from build123d import *

# Parameters (mm, degrees)
CROQUIS1_W                                           = 98
CROQUIS1_H                                           = 80
SALIENTE_EXTRUIR1_DEPTH                              = 200
VACIADO1_T                                           = -5
REDONDEO1_R                                          = 2
CROQUIS6_R                                           = 4.5
CORTAR_EXTRUIR3_DEPTH                                = 401.03249868
REFRENTADO_PARA_TORNILLO_CON_CABEZA_PLAN_D           = 3.4
REFRENTADO_PARA_TORNILLO_CON_CABEZA_PLAN_DEPTH       = 5
REFRENTADO_PARA_TORNILLO_CON_CABEZA_PLAN_CBORE_D     = 6.5
REFRENTADO_PARA_TORNILLO_CON_CABEZA_PLAN_CBORE_DEPTH = 2
CORTAR_EXTRUIR5_REACH                                = 228.283
CROQUIS11_R                                          = 6.5
SIMETR_A3_AT_THE_SECOND_PLANE_COPY_1_REACH           = 228.283
SIMETR_A3_AT_THE_SECOND_PLANE_COPY_1_SKE_R           = 6.5
REFRENTADO_PARA_TORNILLO_CON_CABEZA_2_D              = 3.4
REFRENTADO_PARA_TORNILLO_CON_CABEZA_2_DEPTH          = 5
REFRENTADO_PARA_TORNILLO_CON_CABEZA_2_CBORE_D        = 6.5
REFRENTADO_PARA_TORNILLO_CON_CABEZA_2_CBORE_DEPTH    = 2
REFRENTADO_PARA_TORNILLO_CON_CABEZA_3_D              = 3.4
REFRENTADO_PARA_TORNILLO_CON_CABEZA_3_DEPTH          = 5
REFRENTADO_PARA_TORNILLO_CON_CABEZA_3_CBORE_D        = 6.5
REFRENTADO_PARA_TORNILLO_CON_CABEZA_3_CBORE_DEPTH    = 2
REFRENTADO_PARA_TORNILLO_CON_CABEZA_4_D              = 3.2
REFRENTADO_PARA_TORNILLO_CON_CABEZA_4_DEPTH          = 5
REFRENTADO_PARA_TORNILLO_CON_CABEZA_4_CBORE_D        = 6.5
REFRENTADO_PARA_TORNILLO_CON_CABEZA_4_CBORE_DEPTH    = 2
CROQUIS21_W                                          = 20.5
CROQUIS21_H                                          = 41
CORTAR_EXTRUIR6_DEPTH                                = 10
SALIENTE_EXTRUIR2_DEPTH                              = 42.5
CORTAR_EXTRUIR7_REACH                                = 222.909
CROQUIS24_W                                          = 85
CROQUIS24_H                                          = 221.577794898
SALIENTE_EXTRUIR7_DEPTH                              = 4
CORTAR_EXTRUIR8_REACH                                = 230.263
TALADRO_DE_MARGEN_PARA_M31_D                         = 3.4
TALADRO_DE_MARGEN_PARA_M31_DEPTH                     = 5
TALADRO_DE_MARGEN_PARA_M51_D                         = 5.5
TALADRO_DE_MARGEN_PARA_M51_DEPTH                     = 5
CROQUIS30_W                                          = 10
CROQUIS30_H                                          = 10
SALIENTE_EXTRUIR8_DEPTH                              = 5
TALADRO_DE_MARGEN_PARA_M52_D                         = 5.5
TALADRO_DE_MARGEN_PARA_M52_DEPTH                     = 5


with BuildPart() as part:
    # Croquis1 → Saliente-Extruir1 (new, symmetric)
    with BuildSketch(Plane.XY):
        Rectangle(CROQUIS1_W, CROQUIS1_H)
    extrude(amount=SALIENTE_EXTRUIR1_DEPTH, both=True)

    # Vaciado1
    vaciado1_openings = [part.faces().sort_by_distance(p)[0] for p in [
        (0, 40, 0),
    ]]
    offset(amount=VACIADO1_T, openings=vaciado1_openings, kind=Kind.INTERSECTION)

    # Redondeo1
    redondeo1_edges = [part.edges().sort_by_distance(p)[0] for p in [
        (49, 0, 200),
        (0, -35, -195),
        (0, -35, 195),
        (-49, 0, 200),
        (49, 0, -200),
        (0, -40, -200),
        (-49, 0, -200),
        (49, 40, 0),
        (49, -40, 0),
        (-49, -40, 0),
        (0, -40, 200),
    ]]
    fillet(redondeo1_edges, radius=REDONDEO1_R)

    # Croquis6 → Cortar-Extruir3 (cut, through all)
    with BuildSketch(Plane(origin=(0, 0, 195), x_dir=(-1, 0, 0), z_dir=(0, 0, -1))):
        with Locations((1, 20)):
            Circle(CROQUIS6_R)
    extrude(amount=-CORTAR_EXTRUIR3_DEPTH, mode=Mode.SUBTRACT)

    # Refrentado para tornillo con cabeza plan
    with Locations(Plane.ZY.offset(49)):
        with Locations((-184, -27.06), (-184, -9.06), (-151, -9.06), (-151, -27.06)):
            CounterBoreHole(REFRENTADO_PARA_TORNILLO_CON_CABEZA_PLAN_D / 2, REFRENTADO_PARA_TORNILLO_CON_CABEZA_PLAN_CBORE_D / 2, REFRENTADO_PARA_TORNILLO_CON_CABEZA_PLAN_CBORE_DEPTH, depth=REFRENTADO_PARA_TORNILLO_CON_CABEZA_PLAN_DEPTH)

    # Croquis11 → Cortar-Extruir5 (cut, up to next)
    with BuildSketch(Plane.ZY.offset(49), mode=Mode.PRIVATE) as cortar_extruir5_sk1:
        with Locations(Location((-175, -17.06, 0), (0, 0, 270))):
            Circle(CROQUIS11_R)
    cortar_extruir5_tool1 = extrude(cortar_extruir5_sk1.sketch, amount=-CORTAR_EXTRUIR5_REACH, mode=Mode.PRIVATE) & part.part
    cortar_extruir5 = cortar_extruir5_tool1.solids().sort_by_distance((-49, -17.06, -175))[0]
    add(cortar_extruir5, mode=Mode.SUBTRACT)

    # Simetría3: Cortar-Extruir5 across plane
    add(cortar_extruir5.mirror(Plane.XY), mode=Mode.SUBTRACT)

    # Simetría3 at the second plane: Cortar-Extruir5 across plane
    add(cortar_extruir5.mirror(Plane(origin=(0, 0, 0), x_dir=(0, 0, 1), z_dir=(1, 0, 0))), mode=Mode.SUBTRACT)

    # Simetría3 at the second plane copy 1 ske → Simetría3 at the second plane copy 1 (cut, up to next)
    with BuildSketch(Plane(origin=(49, 0, 0), x_dir=(0, 0, -1), z_dir=(1, 0, 0)), mode=Mode.PRIVATE) as simetr_a3_at_the_second_plane_copy_1_sk1:
        with Locations(Location((-175, -17.06, 0), (0, 0, 270))):
            Circle(SIMETR_A3_AT_THE_SECOND_PLANE_COPY_1_SKE_R)
    simetr_a3_at_the_second_plane_copy_1_tool1 = extrude(simetr_a3_at_the_second_plane_copy_1_sk1.sketch, amount=-SIMETR_A3_AT_THE_SECOND_PLANE_COPY_1_REACH, mode=Mode.PRIVATE) & part.part
    add(simetr_a3_at_the_second_plane_copy_1_tool1.solids().sort_by_distance((49, -17.06, 175))[0], mode=Mode.SUBTRACT)

    # Refrentado para tornillo con cabeza  2
    with Locations(Plane.ZY.offset(49)):
        with Locations((151, -25.06), (151, -7.06), (184, -7.06), (184, -25.06)):
            CounterBoreHole(REFRENTADO_PARA_TORNILLO_CON_CABEZA_2_D / 2, REFRENTADO_PARA_TORNILLO_CON_CABEZA_2_CBORE_D / 2, REFRENTADO_PARA_TORNILLO_CON_CABEZA_2_CBORE_DEPTH, depth=REFRENTADO_PARA_TORNILLO_CON_CABEZA_2_DEPTH)

    # Refrentado para tornillo con cabeza  3
    with Locations(Plane(origin=(49, 0, 0), x_dir=(0, 0, -1), z_dir=(1, 0, 0))):
        with Locations((-151, -9.06), (-184, -9.06), (-184, -27.06), (-151, -27.06)):
            CounterBoreHole(REFRENTADO_PARA_TORNILLO_CON_CABEZA_3_D / 2, REFRENTADO_PARA_TORNILLO_CON_CABEZA_3_CBORE_D / 2, REFRENTADO_PARA_TORNILLO_CON_CABEZA_3_CBORE_DEPTH, depth=REFRENTADO_PARA_TORNILLO_CON_CABEZA_3_DEPTH)

    # Refrentado para tornillo con cabeza  4
    with Locations(Plane(origin=(49, 0, 0), x_dir=(0, 0, -1), z_dir=(1, 0, 0))):
        with Locations((151, -25.06), (151, -7.06), (184, -7.06), (184, -25.06)):
            CounterBoreHole(REFRENTADO_PARA_TORNILLO_CON_CABEZA_4_D / 2, REFRENTADO_PARA_TORNILLO_CON_CABEZA_4_CBORE_D / 2, REFRENTADO_PARA_TORNILLO_CON_CABEZA_4_CBORE_DEPTH, depth=REFRENTADO_PARA_TORNILLO_CON_CABEZA_4_DEPTH)

    # Croquis21 → Cortar-Extruir6 (cut)
    with BuildSketch(Plane(origin=(0, 0, -200), x_dir=(-1, 0, 0), z_dir=(0, 0, -1))):
        with Locations((0, -6.5)):
            Rectangle(CROQUIS21_W, CROQUIS21_H)
    extrude(amount=-CORTAR_EXTRUIR6_DEPTH, mode=Mode.SUBTRACT)

    # Croquis23 → Saliente-Extruir2 (add, symmetric)
    with BuildSketch(Plane(origin=(0, 0, 0), x_dir=(0, 0, -1), z_dir=(1, 0, 0))):
        Polygon((-118, -40), (-103, -50), (103, -50), (118, -40), (110.788897449, -40), (101.788897449, -46), (-101.788897449, -46), (-110.788897449, -40), align=None)
    extrude(amount=SALIENTE_EXTRUIR2_DEPTH, both=True)

    # Croquis24 → Cortar-Extruir7 (cut, up to next)
    with BuildSketch(Plane.XZ.offset(40), mode=Mode.PRIVATE) as cortar_extruir7_sk1:
        Rectangle(CROQUIS24_W, CROQUIS24_H)
    cortar_extruir7_tool1 = extrude(cortar_extruir7_sk1.sketch, amount=-CORTAR_EXTRUIR7_REACH, mode=Mode.PRIVATE) & part.part
    add(cortar_extruir7_tool1.solids().sort_by_distance((0, -40, 0))[0], mode=Mode.SUBTRACT)

    # Croquis25 → Saliente-Extruir7 (add)
    with BuildSketch(Plane(origin=(42.5, 0, 0), x_dir=(0, 0, -1), z_dir=(1, 0, 0))):
        Polygon((103, -50), (118, -40), (-118, -40), (-103, -50), align=None)
    saliente_extruir7 = extrude(amount=SALIENTE_EXTRUIR7_DEPTH)

    # Simetría4: Saliente-Extruir7 across plane
    add(saliente_extruir7.mirror(Plane(origin=(0, 0, 0), x_dir=(0, 0, 1), z_dir=(1, 0, 0))))

    # Croquis26 → Cortar-Extruir8 (cut, up to next)
    with BuildSketch(Plane.ZY.offset(49), mode=Mode.PRIVATE) as cortar_extruir8_sk1:
        with BuildLine():
            Line((-72.325, -8.7), (-72.325, -18.3))
            ThreePointArc((-72.325, -18.3), (-72.032106781, -19.007106781), (-71.325, -19.3))
            Line((-71.325, -19.3), (-56.525, -19.3))
            ThreePointArc((-56.525, -19.3), (-54.403679656, -18.421320344), (-53.525, -16.3))
            Line((-53.525, -16.3), (-53.525, -10.7))
            ThreePointArc((-53.525, -10.7), (-54.403679656, -8.578679656), (-56.525, -7.7))
            Line((-56.525, -7.7), (-71.325, -7.7))
            ThreePointArc((-71.325, -7.7), (-72.032106781, -7.992893219), (-72.325, -8.7))
        make_face()
    cortar_extruir8_tool1 = extrude(cortar_extruir8_sk1.sketch, amount=-CORTAR_EXTRUIR8_REACH, mode=Mode.PRIVATE) & part.part
    add(cortar_extruir8_tool1.solids().sort_by_distance((-49, -13.5, -63.064313))[0], mode=Mode.SUBTRACT)

    # Taladro de margen para M31
    with Locations(Plane.ZY.offset(49)):
        with Locations((-50.425, -13.5), (-75.425, -13.5)):
            Hole(TALADRO_DE_MARGEN_PARA_M31_D / 2, depth=TALADRO_DE_MARGEN_PARA_M31_DEPTH)

    # Taladro de margen para M51
    with Locations(Plane(origin=(0, 0, -200), x_dir=(-1, 0, 0), z_dir=(0, 0, -1))):
        with Locations((-34.833889062, 27.708126477), (0, 0), (34.833889062, 27.708126477), (33.315182526, -29.997125083), (-33.315182526, -29.997125083)):
            Hole(TALADRO_DE_MARGEN_PARA_M51_D / 2, depth=TALADRO_DE_MARGEN_PARA_M51_DEPTH)

    # Croquis30 → Saliente-Extruir8 (add)
    with BuildSketch(Plane(origin=(0, 40, 0), x_dir=(1, 0, 0), z_dir=(0, 1, 0))):
        with Locations((39, 190)):
            Rectangle(CROQUIS30_W, CROQUIS30_H)
        with Locations((-39, 190)):
            Rectangle(CROQUIS30_W, CROQUIS30_H)
        with Locations((-39, -190)):
            Rectangle(CROQUIS30_W, CROQUIS30_H)
        with Locations((39, -190)):
            Rectangle(CROQUIS30_W, CROQUIS30_H)
        with Locations((39, 0)):
            Rectangle(CROQUIS30_W, CROQUIS30_H)
        with Locations((-39, 0)):
            Rectangle(CROQUIS30_W, CROQUIS30_H)
    extrude(amount=-SALIENTE_EXTRUIR8_DEPTH)

    # Taladro de margen para M52
    with Locations(Plane(origin=(0, 40, 0), x_dir=(1, 0, 0), z_dir=(0, 1, 0))):
        with Locations((-39, -190), (-39, 190), (39, 0), (39, 190), (-39, 0), (39, -190)):
            Hole(TALADRO_DE_MARGEN_PARA_M52_D / 2, depth=TALADRO_DE_MARGEN_PARA_M52_DEPTH)


solid = part.part
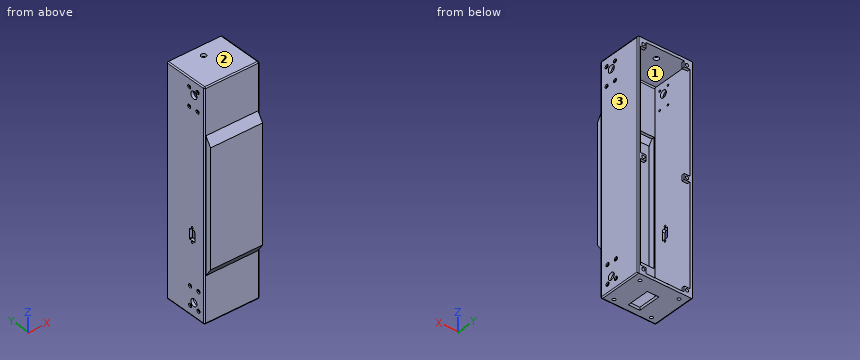
Here's how the part is built. I have some questions about the finished solid (model axes, mm). Face numbers are marked on the shaded views. Round coordinates to 2 decimals unless told otherwise and drop trailing zeros. Order: outer loops, then holes, each group sorted by start corner. A loop starts at its lowest first (then second) coordinate and runs counter-clockwise, first axis right, second up. Notation, with made-up numbers: (68.5, 4) -> (110.5, 4) arc R20 cw to (110.5, 18) -> close; hole circle Ø10 at (47, 61). An arc over 180 degrees is marked (long way). Return JSON: item names as keys, results as strings.
Q1. If we section it at D-D on y = 20: List the corners of the cut face in (x, z) for me, plus the area to 3 significant figures.
Filled sheet:
{"outline": "(-49, -198) arc R2 ccw to (-47, -200) -> (47, -200) arc R2 ccw to (49, -198) -> (49, 198) arc R2 ccw to (47, 200) -> (3.5, 200) -> (3.5, 195) -> (44, 195) -> (44, -195) -> (-44, -195) -> (-44, 195) -> (-5.5, 195) -> (-5.5, 200) -> (-47, 200) arc R2 ccw to (-49, 198) -> close", "area": "4,830 mm^2"}
Q2. If we section it at C-C on x = -1: Give the number of separate pieces and of enclosed holes in the cut face, plus the area to 3 significant figures.
Filled sheet:
{"separate pieces": "3", "enclosed holes": "0", "area": "2,330 mm^2"}
Q3. For pin 1 Ø3 at (y, z) = (-8, -150.5) entering from -X; pin 2 Ø4 at (y, z) = (-9.06, 151) entering from +X; pin 3 Ø5 at (x, z) = (7.5, 83.5) entering from +Y; pin 4 Ø8 at (y, z) = (-17.06, 175) entering from +X, each with a flat end and sliding along its axis, tell me the tip position at first contact or that it passes through.
Filled sheet:
{"pin 1": "stops at x = -47", "pin 2": "stops at x = 47", "pin 3": "stops at y = -46", "pin 4": "passes through"}
Q4. If we section it at B-B on z = -63.5: List the corners of the cut face in (x, y) for me.
Filled sheet:
{"outline": "(-49, -38) arc R2 ccw to (-47, -40) -> (-46.5, -40) -> (-46.5, -50) -> (46.5, -50) -> (46.5, -40) -> (47, -40) arc R2 ccw to (49, -38) -> (49, 38) arc R2 ccw to (47, 40) -> (44, 40) -> (44, -35) -> (42.5, -35) -> (42.5, -46) -> (-42.5, -46) -> (-42.5, -35) -> (-44, -35) -> (-44, -19.3) -> (-49, -19.3) -> close; (-49, -7.7) -> (-44, -7.7) -> (-44, 40) -> (-49, 40) -> close"}
Q5. If we mould it in two halves opening along X, with no side actions, what happens to the marked faces 1, 2 and 3? For each: released by +X, released by -X, zero draft, split by the parting line, or undercut.
Filled sheet:
{"face 1": "undercut", "face 2": "zero draft", "face 3": "released by +X"}
Q6. If we section it at A-A on z = -175: List the corners of the cut face in (x, y) for me, plus the area to 3 significant figures.
Filled sheet:
{"outline": "(-49, -38) arc R2 ccw to (-47, -40) -> (47, -40) arc R2 ccw to (49, -38) -> (49, -23.56) -> (44, -23.56) -> (44, -35) -> (-44, -35) -> (-44, -23.56) -> (-49, -23.56) -> close; (-49, -10.56) -> (-44, -10.56) -> (-44, 40) -> (-49, 40) -> close; (44, -10.56) -> (49, -10.56) -> (49, 38) arc R2 ccw to (47, 40) -> (44, 40) -> close", "area": "1,110 mm^2"}
Q7. I need wall thicknesses on line 1 along Y through (x, z) = (-45.9, -184); line 2 along Z through (x, y) = (-39, 37); line 3 along X through (y, z) = (22, -89.5). Which ranges of each line are inside material? Lowest first, please. Write a range as from..to.
Filled sheet:
{"line 1": "y = -40..-28.76, -25.36..-10.76, -7.36..40", "line 2": "z = -200..-192.75, -187.25..-185, -5..-2.75, 2.75..5, 185..187.25, 192.75..200", "line 3": "x = -49..-44, 44..49"}
